Part model, mm, in its own coordinate system. Face numbers are marked on the shaded views. A direction names the side the tool comes from. Round coordinates to 2 decimals unless told otherwise and drop trailing zeros. Order: outer loops, then holes, each group sorted by start corner. A loop starts at its lowest first (then second) coordinate and runs counter-clockwise, first axis right, second up. Notation, with made-up numbers: (61, -16.5) -> (70, -16.5) arc R34 cw to (70, 14.5) -> close; hole circle Ø8 at (-36, -5). An arc over 180 degrees is marked (long way). Return JSON: item names as keys, results as strings. Group by question number.
from build123d import *

# Parameters (mm, degrees)
F_4_0MM_DOWEL_HOLE2_D               = 4
F_4_0MM_DOWEL_HOLE2_DEPTH           = 8
F_4_0MM_DOWEL_HOLE2_TIP             = 1.201721238
F_4_0MM_DOWEL_HOLE2_ON_FACE_2_D     = 4
F_4_0MM_DOWEL_HOLE2_ON_FACE_2_DEPTH = 8
F_4_0MM_DOWEL_HOLE2_ON_FACE_2_TIP   = 1.201721238
F_4_0MM_DOWEL_HOLE2_ON_FACE_3_D     = 4
F_4_0MM_DOWEL_HOLE2_ON_FACE_3_DEPTH = 8
F_4_0MM_DOWEL_HOLE2_ON_FACE_3_TIP   = 1.201721238
F_4_0MM_DOWEL_HOLE2_ON_FACE_4_D     = 4
F_4_0MM_DOWEL_HOLE2_ON_FACE_4_DEPTH = 8
F_4_0MM_DOWEL_HOLE2_ON_FACE_4_TIP   = 1.201721238
F_6_0MM_DOWEL_HOLE1_D               = 6
F_6_0MM_DOWEL_HOLE1_DEPTH           = 15
F_6_0MM_DOWEL_HOLE1_TIP             = 1.802581857


with BuildPart() as part:
    # Sketch1 → Revolve1 (revolve)
    with BuildSketch(Plane(origin=(0, 0, 0), x_dir=(1, 0, 0), z_dir=(0, 1, 0)), mode=Mode.PRIVATE) as revolve1_sk:
        with BuildLine():
            Line((0, 28), (0, 0))
            Line((0, 0), (24.5618, 0))
            Line((24.5618, 0), (24.5618, 3))
            ThreePointArc((24.5618, 3), (22.5618, 5), (24.5618, 7))
            Line((24.5618, 7), (24.5618, 17))
            ThreePointArc((24.5618, 17), (22.5618, 19), (24.5618, 21))
            Line((24.5618, 21), (24.5618, 24))
            Line((24.5618, 24), (30.099, 24))
            Line((30.099, 24), (30.099, 28))
            Line((30.099, 28), (0, 28))
        make_face()
    revolve(revolve1_sk.sketch.rotate(Axis((0, 0, 0), (0, 0, 1)), 180), axis=Axis((0, 0, 0), (0, 0, 1)))

    # Ø4.0mm Dowel Hole2
    with Locations(Plane(origin=(0, 24.5618, -12), x_dir=(1, 0, 0), z_dir=(0, 1, 0))):
        with Locations((0, 0)):
            Hole(F_4_0MM_DOWEL_HOLE2_D / 2, depth=F_4_0MM_DOWEL_HOLE2_DEPTH)
            with Locations((0, 0, -(F_4_0MM_DOWEL_HOLE2_DEPTH + F_4_0MM_DOWEL_HOLE2_TIP / 2))):  # 118° drill point
                Cone(0, F_4_0MM_DOWEL_HOLE2_D / 2, F_4_0MM_DOWEL_HOLE2_TIP, mode=Mode.SUBTRACT)

    # Ø4.0mm Dowel Hole2 on face 2
    with Locations(Plane(origin=(24.5618, 0, -12), x_dir=(0, 0, 1), z_dir=(1, 0, 0))):
        with Locations((0, 0)):
            Hole(F_4_0MM_DOWEL_HOLE2_ON_FACE_2_D / 2, depth=F_4_0MM_DOWEL_HOLE2_ON_FACE_2_DEPTH)
            with Locations((0, 0, -(F_4_0MM_DOWEL_HOLE2_ON_FACE_2_DEPTH + F_4_0MM_DOWEL_HOLE2_ON_FACE_2_TIP / 2))):  # 118° drill point
                Cone(0, F_4_0MM_DOWEL_HOLE2_ON_FACE_2_D / 2, F_4_0MM_DOWEL_HOLE2_ON_FACE_2_TIP, mode=Mode.SUBTRACT)

    # Ø4.0mm Dowel Hole2 on face 3
    with Locations(Plane(origin=(0, -24.5618, -12), x_dir=(0, 0, -1), z_dir=(0, -1, 0))):
        with Locations((0, 0)):
            Hole(F_4_0MM_DOWEL_HOLE2_ON_FACE_3_D / 2, depth=F_4_0MM_DOWEL_HOLE2_ON_FACE_3_DEPTH)
            with Locations((0, 0, -(F_4_0MM_DOWEL_HOLE2_ON_FACE_3_DEPTH + F_4_0MM_DOWEL_HOLE2_ON_FACE_3_TIP / 2))):  # 118° drill point
                Cone(0, F_4_0MM_DOWEL_HOLE2_ON_FACE_3_D / 2, F_4_0MM_DOWEL_HOLE2_ON_FACE_3_TIP, mode=Mode.SUBTRACT)

    # Ø4.0mm Dowel Hole2 on face 4
    with Locations(Plane(origin=(-24.5618, 0, -12), x_dir=(0, 0, -1), z_dir=(-1, 0, 0))):
        with Locations((0, 0)):
            Hole(F_4_0MM_DOWEL_HOLE2_ON_FACE_4_D / 2, depth=F_4_0MM_DOWEL_HOLE2_ON_FACE_4_DEPTH)
            with Locations((0, 0, -(F_4_0MM_DOWEL_HOLE2_ON_FACE_4_DEPTH + F_4_0MM_DOWEL_HOLE2_ON_FACE_4_TIP / 2))):  # 118° drill point
                Cone(0, F_4_0MM_DOWEL_HOLE2_ON_FACE_4_D / 2, F_4_0MM_DOWEL_HOLE2_ON_FACE_4_TIP, mode=Mode.SUBTRACT)

    # Ø6.0mm Dowel Hole1
    with Locations(Plane(origin=(0, 0, -28), x_dir=(-1, 0, 0), z_dir=(0, 0, -1))):
        with Locations((0, 0)):
            Hole(F_6_0MM_DOWEL_HOLE1_D / 2, depth=F_6_0MM_DOWEL_HOLE1_DEPTH)
            with Locations((0, 0, -(F_6_0MM_DOWEL_HOLE1_DEPTH + F_6_0MM_DOWEL_HOLE1_TIP / 2))):  # 118° drill point
                Cone(0, F_6_0MM_DOWEL_HOLE1_D / 2, F_6_0MM_DOWEL_HOLE1_TIP, mode=Mode.SUBTRACT)


solid = part.part
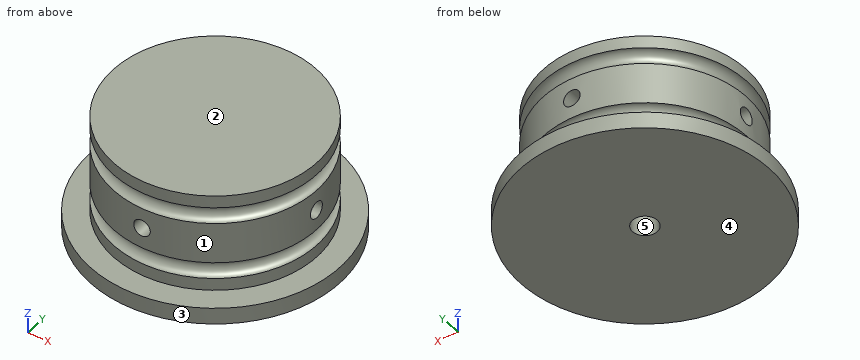
(1) Tool access for the marked faces 1 and 2: list every direction of +Z, -Z, +X, -X, +Y, -Y with a clear straight run to the whole face (end or side of a thin tool).
(2) Mould opens along X. For the marked faces 3, 4 and 5 say: pulls with the +X half, pulls with the -X half, needs draft (parallel to the pull), parting line crosses it, or undercut.
(3) Saw through at C-C, the plane z = -25.25. List the corners of the cut face in (x, y).
(4) Saw through at A-A, the plane z = -15.25. List the corners of the cut face in (x, y).
(5) Probe L1, parallel to Z at x = -21.5, y = 10.5; L2, parallel to Z at x = 0, y = -19.75; L3, parallel to Y at x = 0, z = -23.5. List the from-to ranges inside material, lowest first. Write a range as [from, to].
(6) Saw through at B-B, the plane z = -2. List the corners of the cut face in (x, y), and give its area (3 significant figures).
(7) Pin check, flat tips, straight feed: P1, Ø3.5, axis at x = 0, z = -12, coming from the +Y side; P2, Ø3, axis at x = -16, z = -10.5, coming from the -Y side; P3, Ø3, axis at y = 0, z = -12, coming from the +X side; P4, Ø1, axis at x = -16, y = 6, coming from the +Z side. Stop position of each tip, or through.
Results are:
{
 "1": {"face 1": "+Z", "face 2": "+Z, +X, -X, +Y, -Y"},
 "2": {"face 3": "parting line crosses it", "face 4": "needs draft", "face 5": "undercut"},
 "3": {"outline": "circle Ø60.2 at (0, 0); hole circle Ø6 at (0, 0)"},
 "4": {"outline": "circle Ø49.12 at (0, 0); hole circle Ø6 at (0, 0)"},
 "5": {"L1": "z = [-28, -20.9], [-17.1, -6.9], [-3.1, 0]", "L2": "z = [-28, -14], [-10, 0]", "L3": "y = [-24.56, -3], [3, 24.56]"},
 "6": {"outline": "circle Ø49.12 at (0, 0)", "area": "1,900 mm^2"},
 "7": {"P1": "stops at y = 16.41", "P2": "stops at y = -19.83", "P3": "stops at x = 16.26", "P4": "stops at z = 0"}
}
